from build123d import *

# Parameters (mm, degrees)
BASE_FLANGE1_DEPTH                                   = 60
CSK_FOR_M3_HEX_SOCKET_COUNTERSUNK_CAP_SC_D           = 3.4
CSK_FOR_M3_HEX_SOCKET_COUNTERSUNK_CAP_SC_CSINK_D     = 6.72
CSK_FOR_M3_HEX_SOCKET_COUNTERSUNK_CAP_SC_CSINK_ANGLE = 90
CSK_FOR_M4_COUNTERSUNK_RAISED_HEAD_SCREW_D           = 4.5
CSK_FOR_M4_COUNTERSUNK_RAISED_HEAD_SCREW_CSINK_D     = 9.4
CSK_FOR_M4_COUNTERSUNK_RAISED_HEAD_SCREW_CSINK_ANGLE = 90


# Sheet-metal steps are written as plain solids
with BuildPart() as part:
    # Sketch1 → Base-Flange1 (new body)
    with BuildSketch(Plane.XY):
        with BuildLine():
            Line((-91.244236532, -54.615390039), (46.945285338, -45.450675325))
            ThreePointArc((46.945285338, -45.450675325), (50.13319854, -43.479214131), (50.289406158, -39.734210927))
            Line((50.289406158, -39.734210927), (17.068758356, 29.75632288))
            ThreePointArc((17.068758356, 29.75632288), (16.581579748, 35.359878725), (19.903130417, 39.899094764))
            Line((19.903130417, 39.899094764), (110.167579221, 99.019669419))
            Line((110.167579221, 99.019669419), (112.359212119, 95.673515621))
            Line((112.359212119, 95.673515621), (22.094763314, 36.552940965))
            ThreePointArc((22.094763314, 36.552940965), (20.43398798, 34.283332946), (20.677577284, 31.481555023))
            Line((20.677577284, 31.481555023), (53.898225085, -38.008978784))
            ThreePointArc((53.898225085, -38.008978784), (53.585809851, -45.498985193), (47.209983446, -49.44190758))
            Line((47.209983446, -49.44190758), (-90.979538424, -58.606622294))
            Line((-90.979538424, -58.606622294), (-91.244236532, -54.615390039))
        make_face()
    extrude(amount=BASE_FLANGE1_DEPTH)

    # CSK for M3 Hex Socket Countersunk Cap Screw1 (through all)
    with Locations(Plane(origin=(3.206660902, -48.351416347, 0), x_dir=(0.9978080636970287, 0.06617452698120734, 0), z_dir=(-0.06617452698120732, 0.9978080636970286, 0))):
        with Locations((-56.559497038, -36.126961684)):
            CounterSinkHole(CSK_FOR_M3_HEX_SOCKET_COUNTERSUNK_CAP_SC_D / 2, CSK_FOR_M3_HEX_SOCKET_COUNTERSUNK_CAP_SC_CSINK_D / 2, counter_sink_angle=CSK_FOR_M3_HEX_SOCKET_COUNTERSUNK_CAP_SC_CSINK_ANGLE)

    # CSK for M4 Countersunk Raised Head Screw1 (through all)
    with Locations(Plane(origin=(-10.120981557, 15.452570055, 0), x_dir=(-0.836538449635925, -0.5479082243229453, 0), z_dir=(0.5479082243229453, -0.836538449635925, 0))):
        with Locations((-109.792583779, -36.598273193)):
            CounterSinkHole(CSK_FOR_M4_COUNTERSUNK_RAISED_HEAD_SCREW_D / 2, CSK_FOR_M4_COUNTERSUNK_RAISED_HEAD_SCREW_CSINK_D / 2, counter_sink_angle=CSK_FOR_M4_COUNTERSUNK_RAISED_HEAD_SCREW_CSINK_ANGLE)


solid = part.part
Design review of the part built by this model. Coordinates are the model's own, in mm. A direction names the side the tool comes from. Coordinates: 2 decimals unless noted, no trailing zeros. Loops run counter-clockwise (first coordinate to the right, second up) from the corner with the lowest first, then second, coordinate; pieces in that order, holes last.
Item 1: Draft analysis for pull direction Z (two halves, no side actions). For faces 4 (the cylindrical face through (80.8, 78.9, 38.6)), 5 (the flat face through (-23.117, -50.097, 29.58)), 6 (the conical face through (82.278, 78.758, 37.506)), 7 (the flat face through (34, -3, 60)), state which applies: pulls with the +Z half, pulls with the -Z half, needs draft (parallel to the pull), parting line crosses it, or undercut.
Completed:
face 4: undercut
face 5: needs draft
face 6: undercut
face 7: pulls with the +Z half
Item 2: Add section B-B (z = 45.5). Write out the cut boundary in (x, y), and give its area (3 significant figures).
Completed:
outline: (-91.24, -54.62) - (-90.98, -58.61) - (47.21, -49.44) arc R8 ccw to (53.9, -38.01) - (20.68, 31.48) arc R4 cw to (22.09, 36.55) - (112.36, 95.67) - (110.17, 99.02) - (19.9, 39.9) arc R8 ccw to (17.07, 29.76) - (50.29, -39.73) arc R4 cw to (46.95, -45.45) - close
area: 1,370 mm2
Item 3: Add section C-C (x = -18.5). Write out the cut boundary in (y, z).
Completed:
outline: (-53.8, 0) - (-49.79, 0) - (-49.79, 60) - (-53.8, 60) - close
Item 4: Add section A-A (x = 34). Write out the cut boundary in (y, z), and give its area (3 significant figures).
Completed:
outline: (-50.32, 0) - (-46.31, 0) - (-46.31, 60) - (-50.32, 60) - close; (-5.66, 0) - (3.61, 0) - (3.61, 60) - (-5.66, 60) - close; (44.35, 0) - (49.13, 0) - (49.13, 60) - (44.35, 60) - close
area: 1,080 mm2
Item 5: Clearance check with flat-ended pins moving along their axes: pin 1 (10 mm diameter, centred on x = 20.5, z = 44.5, fed in from +Y); pin 2 (10 mm diameter, centred on y = 13.5, z = 23, fed in from -X); pin 3 (2 mm diameter, centred on x = -57.5, z = 44.5, fed in from -Y). State where each tip first meets the part, or that it passes through.
Completed:
pin 1: stops at y = 43.56
pin 2: stops at x = 22.45
pin 3: stops at y = -56.45
Item 6: For faces 1 (the flat face through (37.055, -2.777, 29.58)), 2 (the flat face through (33.912, -5.475, 29.58)), 3 (the flat face through (34, -3, 0)), list the 3-axis set-ups (+Z, -Z, +X, -X, +Y, -Y) from which the entire face can be reached by the end or side of a thin tool; tool diameter is ignored.
Completed:
face 1: +Z, -Z, +X
face 2: +Z, -Z, -X
face 3: -Z, +X, -X, +Y, -Y
Item 7: Wall thickness on L1, parallel to Y at x = 26, z = 48.5; L2, parallel to Y at x = 40.5, z = 36; L3, parallel to Z at x = 80.5, y = 79: over which ranges is each line inside the solid? List them lowest first.
Completed:
L1: y = -50.85 to -46.84, 11.07 to 20.35, 39.11 to 43.89
L2: y = -49.89 to -45.88, -19.26 to -9.98, 48.61 to 53.39
L3: z = 0 to 34.51, 38.69 to 60
Item 8: Add section D-D (y = 10). Write out the cut boundary in (x, z).
Completed:
outline: (26.51, 0) - (30.95, 0) - (30.95, 60) - (26.51, 60) - close
